Here's how the part is built. I have some questions about the finished solid (model axes, mm). A direction names the side the tool comes from. Coordinates: 2 decimals unless noted, no trailing zeros. Write each loop counter-clockwise with the first axis right and the second up, starting at its lowest first coordinate (ties: lowest second). Pieces come first, ordered by that corner, then holes.
```python
from build123d import *

# Parameters (mm, degrees)
SKETCH1_W          = 82.55
SKETCH1_H          = 76.2
SKETCH1_R          = 28.5877
EXTRUDE1_DEPTH     = 50.8
CUT_EXTRUDE1_DEPTH = 83.55
SKETCH3_R          = 30.988
CUT_EXTRUDE2_DEPTH = 34.925
FILLET1_R          = 1.524
HOLE1_D            = 7.1374
HOLE1_DEPTH        = 76.2


with BuildPart() as part:
    # Sketch1 → Extrude1 (new body)
    with BuildSketch(Plane.XY):
        with Locations((0, 38.1)):
            Rectangle(SKETCH1_W, SKETCH1_H)
        with Locations((0, 38.1)):
            Circle(SKETCH1_R, mode=Mode.SUBTRACT)
    extrude(amount=-EXTRUDE1_DEPTH)

    # Sketch2 → Cut-Extrude1 (cut, through all)
    with BuildSketch(Plane(origin=(41.275, 0, 0), x_dir=(0, 0, -1), z_dir=(1, 0, 0))):
        Polygon((16.002, 76.2), (50.8, 15.748), (50.8, 76.2), align=None)
    extrude(amount=-CUT_EXTRUDE1_DEPTH, mode=Mode.SUBTRACT)

    # Sketch3 → Cut-Extrude2 (cut)
    with BuildSketch(Plane(origin=(0, 0, -50.8), x_dir=(-1, 0, 0), z_dir=(0, 0, -1))):
        with Locations(Location((0, 38.1, 0), (0, 0, 313.83713531))):  # turned: the seam where the file's is
            Circle(SKETCH3_R)
    extrude(amount=-CUT_EXTRUDE2_DEPTH, mode=Mode.SUBTRACT)

    # Fillet1
    fillet1_edges = [part.edges().sort_by_distance(p)[0] for p in [
        (21.462624257, 60.452, -15.875),
    ]]
    fillet(fillet1_edges, radius=FILLET1_R)

    # Hole1
    with Locations(Plane(origin=(0, 76.2, 0), x_dir=(-1, 0, 0), z_dir=(0, 1, 0))):
        with Locations((34.925, -7.874), (-34.925, -7.874)):
            Hole(HOLE1_D / 2, depth=HOLE1_DEPTH)


solid = part.part
```
1) Will this pin go through, and if not, where does the flat tip stop? pin 1 (1 mm diameter, centred on x = 31, z = -24.5, fed in from +Y).
Values follow:
pin 1: stops at y = 62.31
2) Imagine slicing it at D-D on z = -31. Please give me the cut outline in (x, y) (3 decimals), then the cut area to 3 significant figures.
Values follow:
outline: (-41.275, 0) - (41.275, 0) - (41.275, 50.145) - (28.551, 50.145) arc R30.988 cw (long way) to (-28.551, 50.145) - (-41.275, 50.145) - close
area: 1,900 mm2
3) Imagine slicing it at B-B on z = -13. Please give me the cut outline in (x, y) (3 decimals), then the cut area to 3 significant figures.
Values follow:
outline: (-41.275, 0) - (41.275, 0) - (41.275, 76.2) - (-41.275, 76.2) - close; hole circle Ø57.175 at (0, 38.1)
area: 3,720 mm2
4) I need wall thicknesses on probe 1 along X at (y, z) = (61, -11) (3 decimals); probe 2 along X at (y, z) = (71, -10.5) (3 decimals); probe 3 along Z at (x, y) = (-12, 11). Which ranges of each line are inside material? Lowest first, please.
Values follow:
probe 1: x = -41.275 to -36.647, -33.203 to -17.113, 17.113 to 33.203, 36.647 to 41.275
probe 2: x = -41.275 to -37.342, -32.508 to 32.508, 37.342 to 41.275
probe 3: z = -15.88 to 0
5) We'd pull the mould along Z, two halves only. Please class faces 1 (the face through (0.578, 73.265, -17.692)), 2 (the face through (-31.52, 37.57, -6.8)), 3 (the face through (41.275, 29, -19)): pulls with the +Z half, pulls with the -Z half, needs draft (parallel to the pull), parting line crosses it, or undercut.
Values follow:
face 1: pulls with the -Z half
face 2: undercut
face 3: needs draft
6) Imagine slicing it at A-A on y = 38.1. Please give me the cut outline in (x, z) (3 decimals), then the cut area to 3 significant figures.
Values follow:
outline: (-41.275, -37.934) - (-30.988, -37.934) - (-30.988, -17.399) arc R1.524 cw to (-29.464, -15.875) - (-28.588, -15.875) - (-28.588, 0) - (-41.275, 0) - close; (28.588, -15.875) - (29.464, -15.875) arc R1.524 cw to (30.988, -17.399) - (30.988, -37.934) - (41.275, -37.934) - (41.275, 0) - (28.588, 0) - close; hole circle Ø7.137 at (-34.925, -7.874); hole circle Ø7.137 at (34.925, -7.874)
area: 778 mm2
7) Imagine slicing it at C-C on x = 0. Please give me the cut outline in (y, z) (3 decimals), then the cut area to 3 significant figures.
Values follow:
outline: (0, -50.8) - (7.112, -50.8) - (7.112, -17.399) arc R1.524 cw to (8.636, -15.875) - (9.512, -15.875) - (9.512, 0) - (0, 0) - close; (66.688, -15.875) - (67.564, -15.875) arc R1.524 cw to (69.088, -17.399) - (69.088, -20.096) - (76.2, -16.002) - (76.2, 0) - (66.688, 0) - close
area: 567 mm2
8) On a 3-axis mill with a long thin cutter (end or side, diameter ignored), from which of +Z, -Z, +X, -X, +Y, -Y can I reach the whole of each face in a straight line? I mean faces 4 (the face through (-7, 66, -15.875)), 5 (the face through (-1, 6, -50.8)). Say none if no direction works.
Values follow:
face 4: -Z
face 5: -Z, +X, -X, +Y, -Y
